The figure shows three views and two pictorial views of one solid part (mm, origin at its lowest corner). Answer the questions. A direction names the side the tool comes from. Give positions to 0.01 mm unless a question says otherwise; leave off trailing zeros. Write each loop counter-clockwise with the first axis right and the second up, starting at its lowest first coordinate (ties: lowest second). Pieces come first, ordered by that corner, then holes. Notation, with made-up numbers: (16.5, -31.5) - (50.5, -31.5) arc R22 ccw to (50.5, -3.5) - close; hole circle Ø2 at (22.5, 67). An arc over 180 degrees is marked (long way). Use CSV: the item, a comma, the result in double quotes. Start each with the question number.
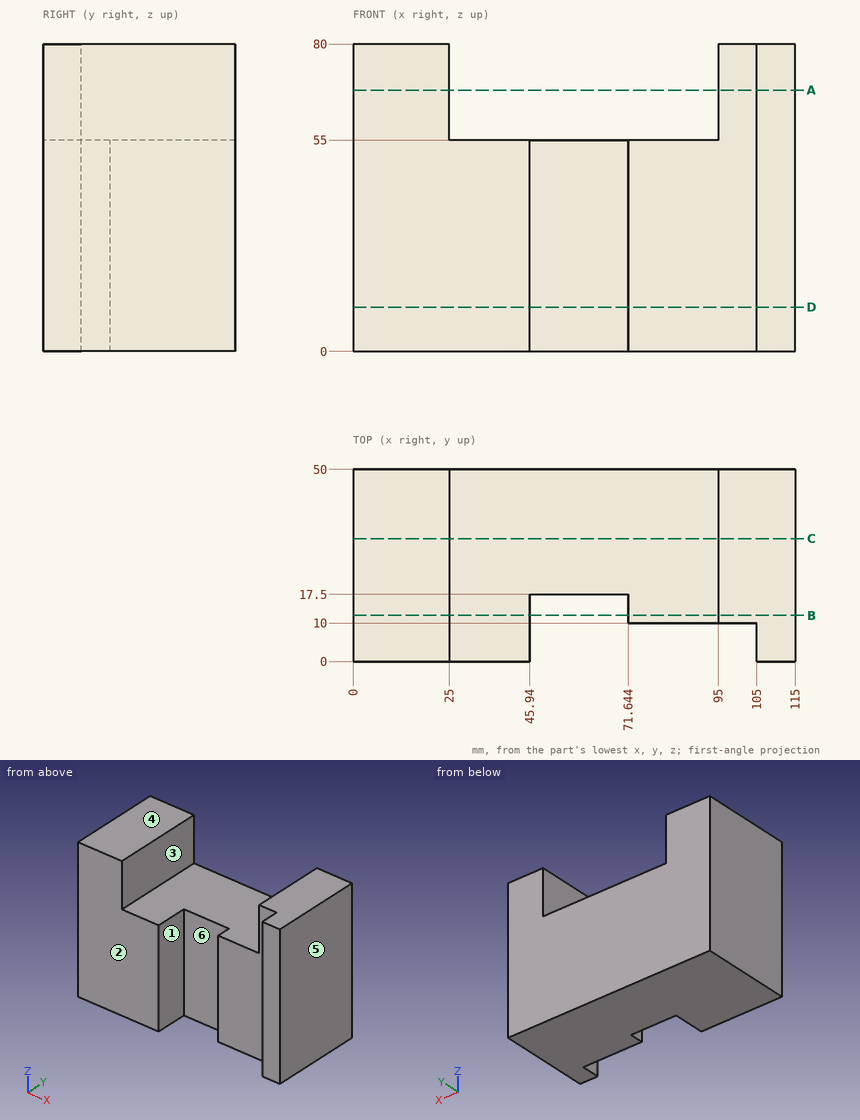
(1) Given P1, Ø8, axis at x = 31, y = 39.5, coming from the -Z side; P2, Ø13, axis at x = 57.5, z = 39.5, coming from the -Y side; P3, Ø3, axis at x = 44, y = 21.5, coming from the +Z side, each flat-ended and moving along its own axis, determine where each tip first touches the part or whether it passes through.
(2) The part is cut by section B-B on y = 12. Write down the section's boundary in (x, z), plus the area to 3 significant figures.
(3) Consider probe 1 along X at (y, z) = (21, 77); probe 2 along X at (y, z) = (5.5, 47); probe 3 along Z at (x, y) = (39.5, 14). Determine where each line is inside the solid, lowest interval first.
(4) The part is cut by section A-A on z = 68. Write down the section's boundary in (x, y).
(5) The part is cut by section C-C on y = 32. Write down the section's boundary in (x, z).
(6) The part is cut by section D-D on z = 11.5. Write down the section's boundary in (x, y).
(7) Which of the six approach directions +Z, -Z, +X, -X, +Y, -Y give full straight-line access (tool end or side, diameter ignored) to the marked faces 1, 2 and 3?
(8) For a pull along X with two mould halves and no side action, classify the marked faces 4, 5 and 6 as pulls with the +X half, pulls with the -X half, needs draft (parallel to the pull), parting line crosses it, or undercut.
Reported:
1,P1,"z = 0"
1,P2,"y = 17.5"
1,P3,"z = 55"
2,outline,"(0, 0) - (45.94, 0) - (45.94, 55) - (25, 55) - (25, 80) - (0, 80) - close; (71.64, 0) - (115, 0) - (115, 80) - (95, 80) - (95, 55) - (71.64, 55) - close"
2,area,"6,040 mm²"
3,probe 1,"0 to 25, 95 to 115"
3,probe 2,"0 to 45.94, 105 to 115"
3,probe 3,"0 to 55"
4,outline,"(0, 0) - (25, 0) - (25, 50) - (0, 50) - close; (95, 10) - (105, 10) - (105, 0) - (115, 0) - (115, 50) - (95, 50) - close"
5,outline,"(0, 0) - (115, 0) - (115, 80) - (95, 80) - (95, 55) - (25, 55) - (25, 80) - (0, 80) - close"
6,outline,"(0, 0) - (45.94, 0) - (45.94, 17.5) - (71.64, 17.5) - (71.64, 10) - (105, 10) - (105, 0) - (115, 0) - (115, 50) - (0, 50) - close"
7,face 1,"+Z, -Z, -Y"
7,face 2,"+Z, -Z, +X, -X, -Y"
7,face 3,"+Z, +Y, -Y"
8,face 4,"needs draft"
8,face 5,"pulls with the +X half"
8,face 6,"undercut"
